Input: dimensioned drawing with shaded views. Units: mm. Origin: part minimum x, y, z. Give positions to 0.01 mm unless a question says otherwise; leave off trailing zeros. Order: outer loops, then holes, each group sorted by start corner. A loop starts at its lowest first (then second) coordinate and runs counter-clockwise, first axis right, second up. Notation, with made-up numbers: (73, -35) - (109, -35) arc R19 ccw to (109, -20) - close; hole circle Ø9 at (30, 34). An arc over 180 degrees is marked (long way). Use a Markdown table: item, result.
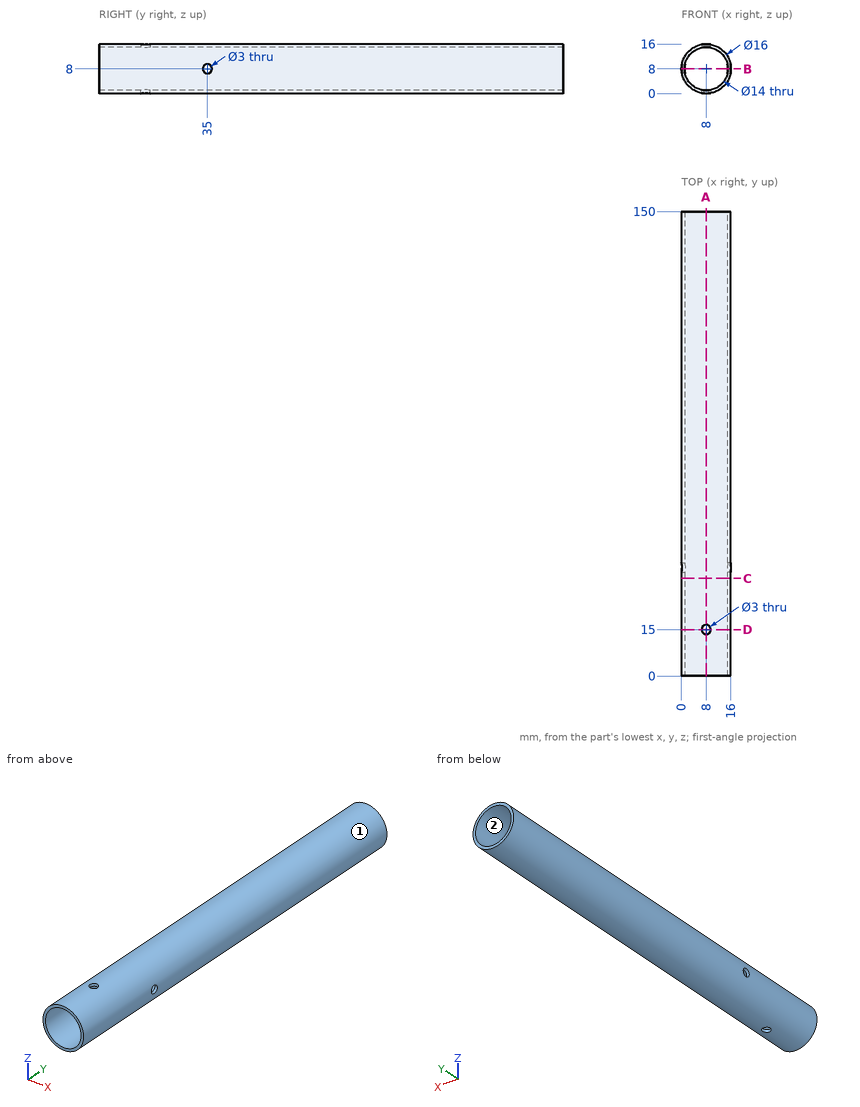
1. Pin query (flat end, axial travel): pin 1 (1.5 mm diameter, centred on x = 12, y = 19, fed in from -Z); pin 2 (1.5 mm diameter, centred on x = 5, y = 49.5, fed in from +Z); pin 3 (3 mm diameter, centred on x = 2.5, y = 64, fed in from +Z). Return the tip coordinate at first contact, or that it passes through.
Response:
| item | result |
|---|---|
| pin 1 | stops at z = 0.69 |
| pin 2 | stops at z = 15.68 |
| pin 3 | stops at z = 14.93 |
2. Section query B-B (z = 8). Return loops of the section in (x, y).
Response:
| item | result |
|---|---|
| outline | (0, 0) - (1, 0) - (1, 33.5) - (0, 33.5) - close; (0, 36.5) - (1, 36.5) - (1, 150) - (0, 150) - close; (15, 0) - (16, 0) - (16, 33.5) - (15, 33.5) - close; (15, 36.5) - (16, 36.5) - (16, 150) - (15, 150) - close |
3. Section query D-D (y = 15). Return loops of the section in (x, z).
Response:
| item | result |
|---|---|
| outline | (6.5, 0.14) - (6.5, 1.16) arc R7 cw to (6.5, 14.84) - (6.5, 15.86) arc R8 ccw to start; (9.5, 0.14) arc R8 ccw to (9.5, 15.86) - (9.5, 14.84) arc R7 cw to (9.5, 1.16) - close |
4. Mould query, pull axis Z, two halves, no side actions, for the marked faces 1 and 2. Classes: pulls with the +Z half, pulls with the -Z half, needs draft (parallel to the pull), parting line crosses it, or undercut.
Response:
| item | result |
|---|---|
| face 1 | parting line crosses it |
| face 2 | undercut |
5. Section query A-A (x = 8). Return loops of the section in (y, z), then the cut area to 3 significant figures.
Response:
| item | result |
|---|---|
| outline | (0, 0) - (13.5, 0) - (13.5, 1) - (0, 1) - close; (0, 15) - (13.5, 15) - (13.5, 16) - (0, 16) - close; (16.5, 0) - (150, 0) - (150, 1) - (16.5, 1) - close; (16.5, 15) - (150, 15) - (150, 16) - (16.5, 16) - close |
| area | 294 mm^2 |
6. Section query C-C (y = 31.5). Return loops of the section in (x, z).
Response:
| item | result |
|---|---|
| outline | circle Ø16 at (8, 8); hole circle Ø14 at (8, 8) |
7. Material intervals for line 1 along Z through (x, y) = (8, 39.5); line 2 along Y through (x, z) = (8, 0.65); line 3 along Z through (x, y) = (14, 13), sorted ascending.
Response:
| item | result |
|---|---|
| line 1 | z = 0 to 1, 15 to 16 |
| line 2 | y = 0 to 13.5, 16.5 to 150 |
| line 3 | z = 2.71 to 4.39, 11.61 to 13.29 |
